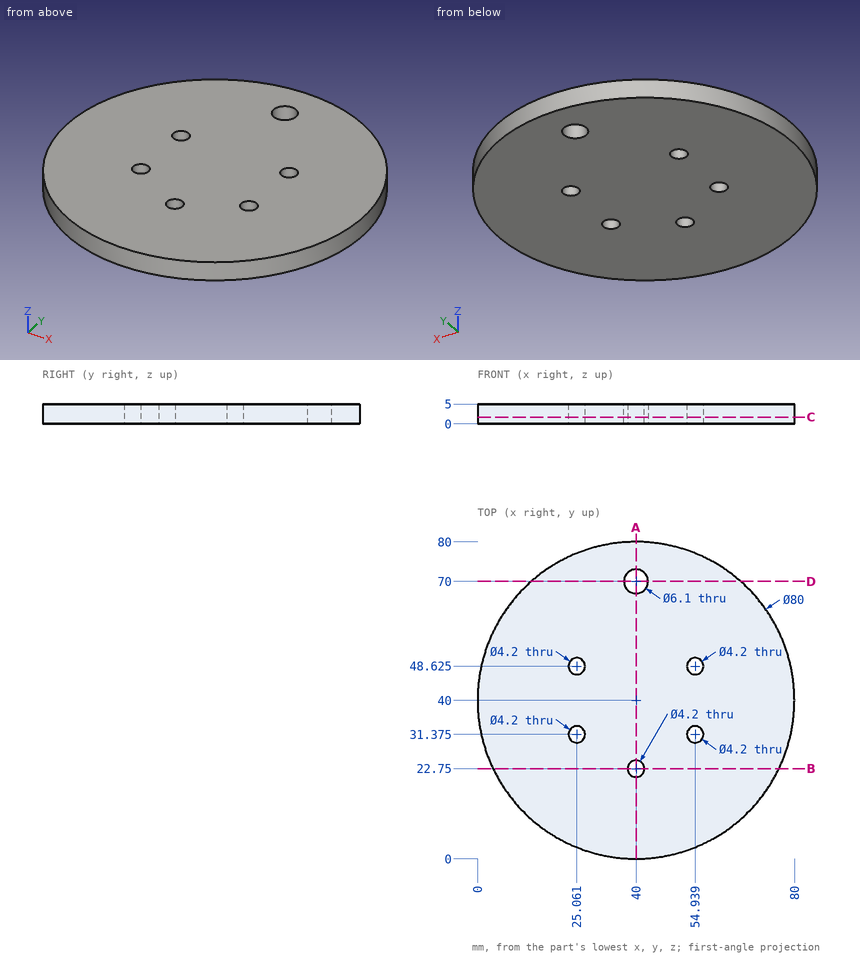
Part print with two shaded views. Sizes in mm from the minimum x, y, z corner. Round coordinates to 2 decimals unless told otherwise and drop trailing zeros. Order: outer loops, then holes, each group sorted by start corner. A loop starts at its lowest first (then second) coordinate and runs counter-clockwise, first axis right, second up. Notation, with made-up numbers: M -3,43.25 L 48,43.25 A32 cw 48,80.25 Z; hole C 56.5,70 d5. An arc over 180 degrees is marked long. Answer in a Markdown table with one row per item. Add a question column.
Q1. Pin check, flat tips, straight feed: pin 1 (3.5 mm diameter, centred on x = 25.06, y = 31.38, fed in from -Z); pin 2 (2 mm diameter, centred on x = 61.5, z = 4, fed in from -Y). Stop position of each tip, or through.
Q2. Cut at D-D on y = 70. Give the cut face in (x, z), and give its area (3 significant figures).
Q3. Cut at C-C on z = 1.7. Give the cut face in (x, y) (3 decimals).
Q4. Cut at B-B on y = 22.75. Give the cut face in (x, z).
Q5. Wall check: L1, parallel to Y at x = 40, z = 3.55; L2, parallel to X at y = 30, z = 0.75; L3, parallel to X at y = 33, z = 0.7. Give the ranges that are in metal, low to high. Write a range as from..to.
Q6. Cut at A-A on x = 40. Give the cut face in (y, z), and give its area (4 significant figures).
Established:
| question | item | result |
|---|---|---|
| 1 | pin 1 | passes through |
| 1 | pin 2 | stops at y = 5.65 |
| 2 | outline | M 13.54,0 L 36.95,0 L 36.95,5 L 13.54,5 Z; M 43.05,0 L 66.46,0 L 66.46,5 L 43.05,5 Z |
| 2 | area | 234 mm2 |
| 3 | outline | C 40,40 d80; hole C 25.061,31.375 d4.2; hole C 25.061,48.625 d4.2; hole C 40,70 d6.1; hole C 40,22.75 d4.2; hole C 54.939,31.375 d4.2; hole C 54.939,48.625 d4.2 |
| 4 | outline | M 3.91,0 L 37.9,0 L 37.9,5 L 3.91,5 Z; M 42.1,0 L 76.09,0 L 76.09,5 L 42.1,5 Z |
| 5 | L1 | y = 0..20.65, 24.85..66.95, 73.05..80 |
| 5 | L2 | x = 1.27..23.47, 26.65..53.35, 56.53..78.73 |
| 5 | L3 | x = 0.62..23.73, 26.39..53.61, 56.27..79.38 |
| 6 | outline | M 0,0 L 20.65,0 L 20.65,5 L 0,5 Z; M 24.85,0 L 66.95,0 L 66.95,5 L 24.85,5 Z; M 73.05,0 L 80,0 L 80,5 L 73.05,5 Z |
| 6 | area | 348.5 mm2 |
